Geometry check sheet. Reference: the model listing, model coordinates, mm. A direction names the side the tool comes from. Give positions to 0.01 mm unless a question says otherwise; leave off trailing zeros. Loops run counter-clockwise (first coordinate to the right, second up) from the corner with the lowest first, then second, coordinate; pieces in that order, holes last. Notation, with made-up numbers: (58, 29.5) -> (74, 29.5) arc R17 cw to (74, 50.5) -> close; hole circle Ø7 at (-36, 48). An arc over 180 degrees is marked (long way). Write item = value, one per line. Start each with the question number.
```python
from build123d import *

# Parameters (mm, degrees)
SKETCH1_W           = 550
SKETCH1_H           = 20
SKETCH1_R           = 5
BOSS_EXTRUDE1_DEPTH = 30
SKETCH3_W           = 25
SKETCH3_H           = 5
CUT_EXTRUDE2_DEPTH  = 552.180551181


with BuildPart() as part:
    # Sketch1 → Boss-Extrude1 (new body)
    with BuildSketch(Plane.XY):
        with Locations((275, 10)):
            Rectangle(SKETCH1_W, SKETCH1_H)
        with Locations((10, 10)):
            Circle(SKETCH1_R, mode=Mode.SUBTRACT)
        with Locations((543, 10)):
            Circle(SKETCH1_R, mode=Mode.SUBTRACT)
    extrude(amount=-BOSS_EXTRUDE1_DEPTH)

    # Sketch3 → Cut-Extrude2 (cut, through all)
    with BuildSketch(Plane(origin=(0, 20, 0), x_dir=(1, 0, 0), z_dir=(0, 1, 0))):
        with Locations((537.5, 2.5)):
            Rectangle(SKETCH3_W, SKETCH3_H)
        with Locations((537.5, 27.5)):
            Rectangle(SKETCH3_W, SKETCH3_H)
    extrude(amount=-CUT_EXTRUDE2_DEPTH, mode=Mode.SUBTRACT)


solid = part.part
```
1) Depth check by flat-ended pin: pin 1 Ø8 at (x, z) = (425.5, -12) entering from -Y; pin 2 Ø6 at (x, y) = (10, 10) entering from -Z; pin 3 Ø10 at (x, y) = (537.5, 13.5) entering from -Z. Enter the tip coordinate at first touch or a pass-through.
2) Section check C-C (x = 543). Enter the section's corners in (y, z), plus the area to 3 significant figures.
3) Thickness scan on line 1 (X direction, y = 9.5, z = -21.25); line 2 (X direction, y = 6.75, z = -12.25); line 3 (Y direction, x = 10, z = -13.5). Record the ranges inside material, lowest first.
4) Section check B-B (x = 10). Enter the section's corners in (y, z), plus the area to 3 significant figures.
5) Section check A-A (y = 10). Enter the section's corners in (x, z).
6) Tool access check on faces 4 (the flat face through (537, 10, -5)), 5 (the flat face through (259, 10, -30)), 6 (the flat face through (537, 10, -25)). Record the directions out of +Z, -Z, +X, -X, +Y, -Y that give a thin tool (end or side, any length) a straight path to the whole face; none if there is none.
7) Draft check along Y on faces 1 (the cylindrical face through (547.619, 8.085, -14.86)), 2 (the flat face through (271, 0, -15)), 3 (the flat face through (0, 10, -15)). Enter one of: released by +Y, released by -Y, zero draft, split by the parting line, or undercut.
Check result:
q1.pin_1 = 0
q1.pin_2 = through
q1.pin_3 = -25
q2.outline = (0, -25) -> (5, -25) -> (5, -5) -> (0, -5) -> close; (15, -25) -> (20, -25) -> (20, -5) -> (15, -5) -> close
q2.area = 200 mm2
q3.line_1 = 0 to 5.03, 14.97 to 538.03, 547.97 to 550
q3.line_2 = 0 to 6.2, 13.8 to 539.2, 546.8 to 550
q3.line_3 = 0 to 5, 15 to 20
q4.outline = (0, -30) -> (5, -30) -> (5, 0) -> (0, 0) -> close; (15, -30) -> (20, -30) -> (20, 0) -> (15, 0) -> close
q4.area = 300 mm2
q5.outline = (0, -30) -> (5, -30) -> (5, 0) -> (0, 0) -> close; (15, -30) -> (525, -30) -> (525, -25) -> (538, -25) -> (538, -5) -> (525, -5) -> (525, 0) -> (15, 0) -> close; (548, -25) -> (550, -25) -> (550, -5) -> (548, -5) -> close
q6.face_4 = +Z, +X, +Y, -Y
q6.face_5 = -Z, +X, -X, +Y, -Y
q6.face_6 = -Z, +X, +Y, -Y
q7.face_1 = undercut
q7.face_2 = released by -Y
q7.face_3 = zero draft
